The drawing under review shows one solid part. Ordinate dimensions are in mm from its lowest x, y, z. Coordinates: 2 decimals unless noted, no trailing zeros. Loops run counter-clockwise (first coordinate to the right, second up) from the corner with the lowest first, then second, coordinate; pieces in that order, holes last. Notation, with made-up numbers: M 73,82.5 L 131,82.5 A24 ccw 131,100.5 Z; hole C 13.5,-36.75 d10. An arc over 180 degrees is marked long. Use one line per item in the form item = value.
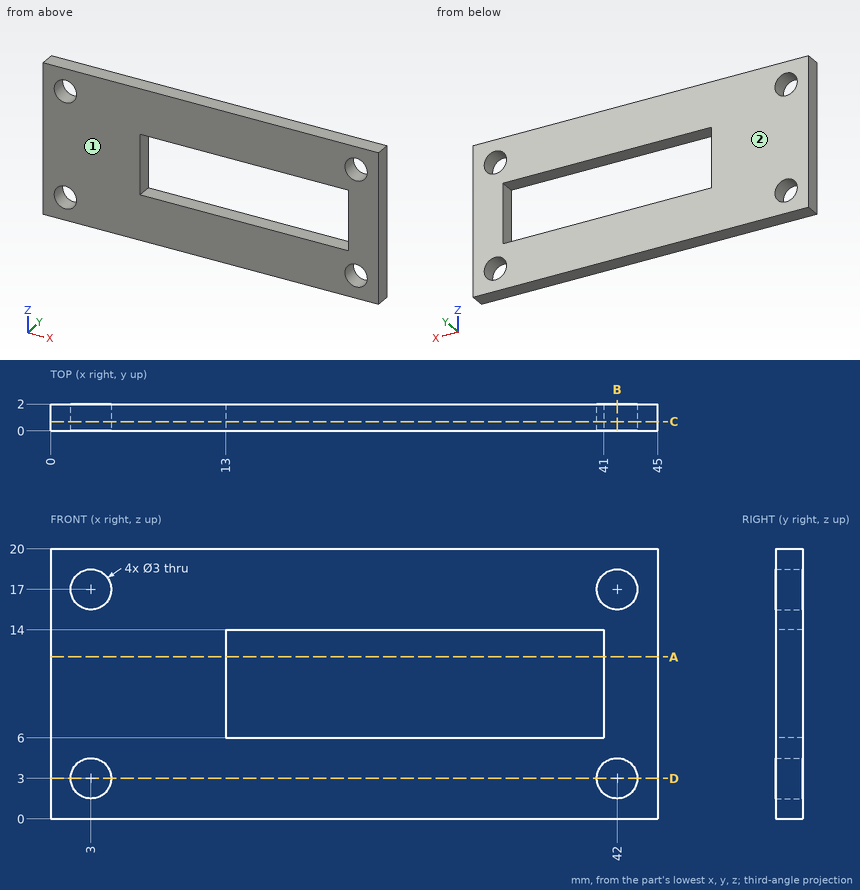
1. Consider section B-B on x = 42. Write out the cut boundary in (y, z), plus the area to 3 significant figures.
Computed values:
outline = M 0,0 L 2,0 L 2,1.5 L 0,1.5 Z; M 0,4.5 L 2,4.5 L 2,15.5 L 0,15.5 Z; M 0,18.5 L 2,18.5 L 2,20 L 0,20 Z
area = 28.0 mm2
2. For pin 1 Ø2.5 at (x, z) = (42, 3) entering from -Y, flat-tipped, find the tip position at first contact; note if it passes through.
Computed values:
pin_1 = through
3. Wall thickness on line 1 along X through (y, z) = (1.1, 17); line 2 along Z through (x, y) = (3, 1.35); line 3 along Z through (x, y) = (25.5, 0.4): over which ranges is each line inside the solid? List them lowest first. Write a range as from..to.
Computed values:
line_1 = 0..1.5, 4.5..40.5, 43.5..45
line_2 = 0..1.5, 4.5..15.5, 18.5..20
line_3 = 0..6, 14..20
4. Consider section A-A on z = 12. Write out the cut boundary in (x, y).
Computed values:
outline = M 0,0 L 13,0 L 13,2 L 0,2 Z; M 41,0 L 45,0 L 45,2 L 41,2 Z
5. Draft analysis for pull direction Y (two halves, no side actions). For the marked faces 1 and 2, state which applies: +Y half, -Y half, draft (parallel to the pull), parting line (faces both ways), or undercut.
Computed values:
face_1 = -Y half
face_2 = +Y half
6. Consider section D-D on z = 3. Write out the cut boundary in (x, y), plus the area to 3 significant figures.
Computed values:
outline = M 0,0 L 1.5,0 L 1.5,2 L 0,2 Z; M 4.5,0 L 40.5,0 L 40.5,2 L 4.5,2 Z; M 43.5,0 L 45,0 L 45,2 L 43.5,2 Z
area = 78.0 mm2
7. Consider section C-C on y = 0.7. Write out the cut boundary in (x, z).
Computed values:
outline = M 0,0 L 45,0 L 45,20 L 0,20 Z; hole C 3,3 d3; hole C 3,17 d3; hole M 13,6 L 41,6 L 41,14 L 13,14 Z; hole C 42,3 d3; hole C 42,17 d3
